Input: part model. Units: mm. Frame: model coordinates. A direction names the side the tool comes from. Round coordinates to 2 decimals unless told otherwise and drop trailing zeros. Loops run counter-clockwise (first coordinate to the right, second up) from the corner with the lowest first, then second, coordinate; pieces in that order, holes last. Notation, with made-up numbers: (4, -28) -> (62, -28) arc R23 ccw to (62, -5) -> close; hole circle Ø3 at (-15.5, 25). An arc over 180 degrees is marked (long way). Answer in a Markdown table with one row per item. Add a question column.
Q1. Section A-A, the plane y = -21. Output: boundary loops of the cut face in (x, z).
Q2. Mould query, pull axis X, two halves, no side actions, for faces 3 (the face through (1, -54, 0)), 4 (the face through (35.871, -78.982, 1.479)), 5 (the face through (-29.65, -36.99, 1.52)), 6 (the face through (-43, -46, 1)). Classes: pulls with the +X half, pulls with the -X half, needs draft (parallel to the pull), parting line crosses it, or undercut.
Q3. Reachability of faces 1 (the face through (32.5, -17, 2)), 2 (the face through (1, -54, 3)) from +Z, -Z, +X, -X, +Y, -Y: full face, straight path, thin tool, end or side. Return the list, or none.
Q4. Section B-B, the plane z = 1.45. Output: boundary loops of the cut face in (x, y).
Q5. Section D-D, the plane x = 1. Output: boundary loops of the cut face in (y, z).
Q6. Pin query (flat end, axial travel): pin 1 (1.5 mm diameter, centred on x = 10.5, z = 1.5, fed in from +Y); pin 2 (1.5 mm diameter, centred on y = -10.5, z = 1, fed in from -X). Return the tip coordinate at first contact, or that it passes through.
Q7. Section C-C, the plane y = -33. Output: boundary loops of the cut face in (x, z), and give its area (3 significant figures).
Q8. Ray query, L1, parallel to Y at x = -10, z = 2.2; L2, parallel to X at y = -14, z = 2.6; L3, parallel to X at y = -28, z = 1.15. Return the intervals inside material, ascending. Write a range as from..to.
```python
from build123d import *

# Parameters (mm, degrees)
BOSS_EXTRUDE1_DEPTH = 3
CUT_EXTRUDE1_DEPTH  = 10


with BuildPart() as part:
    # Sketch1 → Boss-Extrude1 (new body)
    with BuildSketch(Plane.XY):
        with BuildLine():
            Line((-5, 8.5), (5, 8.5))
            ThreePointArc((5, 8.5), (31.870057685, -2.629942315), (43, -29.5))
            Line((43, -29.5), (43, -61.5))
            ThreePointArc((43, -61.5), (35.67766953, -79.17766953), (18, -86.5))
            Line((18, -86.5), (0.5, -86.5))
            Line((0.5, -86.5), (-0.5, -86.5))
            Line((-0.5, -86.5), (-18, -86.5))
            ThreePointArc((-18, -86.5), (-35.67766953, -79.17766953), (-43, -61.5))
            Line((-43, -61.5), (-43, -29.5))
            ThreePointArc((-43, -29.5), (-31.870057685, -2.629942315), (-5, 8.5))
        make_face()
    extrude(amount=BOSS_EXTRUDE1_DEPTH)

    # Sketch2 → Cut-Extrude1 (cut)
    with BuildSketch(Plane.XY.offset(3)):
        with BuildLine():
            Line((-22.5, -40), (22.5, -40))
            ThreePointArc((22.5, -40), (29.571067812, -37.071067812), (32.5, -30))
            Line((32.5, -30), (32.5, 20))
            ThreePointArc((32.5, 20), (29.571067812, 27.071067812), (22.5, 30))
            Line((22.5, 30), (-22.5, 30))
            ThreePointArc((-22.5, 30), (-29.571067812, 27.071067812), (-32.5, 20))
            Line((-32.5, 20), (-32.5, -30))
            ThreePointArc((-32.5, -30), (-29.571067812, -37.071067812), (-22.5, -40))
        make_face()
    extrude(amount=-CUT_EXTRUDE1_DEPTH, mode=Mode.SUBTRACT)


solid = part.part
```
Answer block:
| question | item | result |
|---|---|---|
| 1 | outline | (-42.04, 0) -> (-32.5, 0) -> (-32.5, 3) -> (-42.04, 3) -> close; (32.5, 0) -> (42.04, 0) -> (42.04, 3) -> (32.5, 3) -> close |
| 2 | face 3 | needs draft |
| 2 | face 4 | pulls with the +X half |
| 2 | face 5 | undercut |
| 2 | face 6 | pulls with the -X half |
| 3 | face 1 | +Z, -Z, +Y |
| 3 | face 2 | +Z, +X, -X, +Y, -Y |
| 4 | outline | (-43, -61.5) arc R25 ccw to (-18, -86.5) -> (18, -86.5) arc R25 ccw to (43, -61.5) -> (43, -29.5) arc R38 ccw to (32.5, -3.28) -> (32.5, -30) arc R10 cw to (22.5, -40) -> (-22.5, -40) arc R10 cw to (-32.5, -30) -> (-32.5, -3.28) arc R38 ccw to (-43, -29.5) -> close |
| 5 | outline | (-86.5, 0) -> (-40, 0) -> (-40, 3) -> (-86.5, 3) -> close |
| 6 | pin 1 | y = -40 |
| 6 | pin 2 | x = -38.33 |
| 7 | outline | (-43, 0) -> (-32.04, 0) -> (-32.04, 3) -> (-43, 3) -> close; (32.04, 0) -> (43, 0) -> (43, 3) -> (32.04, 3) -> close |
| 7 | area | 65.8 mm^2 |
| 8 | L1 | -86.5..-40 |
| 8 | L2 | -39.7..-32.5, 32.5..39.7 |
| 8 | L3 | -42.97..-32.5, 32.5..42.97 |
